Can you work these out from the model? Positions are in its coordinate system, mm. Face numbers are marked on the shaded views. A direction names the side the tool comes from. Give positions to 0.01 mm unless a question says otherwise; leave off trailing zeros. Loops run counter-clockwise (first coordinate to the right, second up) from the corner with the lowest first, then second, coordinate; pieces in that order, holes last. Notation, with made-up numbers: (-24, -35.75) -> (-7, -35.75) arc R12 cw to (-7, -25.75) -> close; hole circle Ø1 at (68.25, 38). An arc over 180 degrees is marked (long way). One line per question, with ' | ' between items.
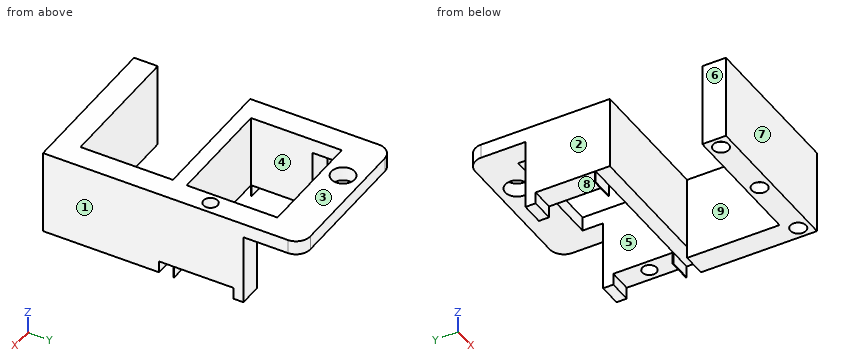
Autodesk Inventor part; units mm, degrees
ref_plane "Work Plane2" through (28, 0, 0) normal (0, 0, 1) x (1, 0, 0)
ref_plane "Work Plane3" through (0, -3.15, -2.5) normal (0, 0, 1) x (1, 0, 0)
ref_plane "YZ Plane" through (0, 0, 0) normal (1, 0, 0) x (0, 1, 0)
ref_plane "Work Plane1" through (5, 0, 4.5) normal (0, 0, 1) x (1, 0, 0)
sketch "Sketch1" plane through (5, 0, 4.5) normal (0, 0, 1) x (1, 0, 0)
  circle A0 centre (25.5, 6.25) radius 1.5
  line L0 (28, 14.65) -> (28, -27.65)
  line L1 (23.15, 14.65) -> (28, 14.65)
  line L2 (23.15, 14.65) -> (23.15, -0.15)
  line L3 (-0.15, -0.15) -> (23.15, -0.15)
  line L4 (-0.15, 14.65) -> (-0.15, -0.15)
  line L5 (-5, 14.65) -> (-0.15, 14.65)
  line L6 (-5, 14.65) -> (-5, -3.15)
  line L7 (23, -3.15) -> (-5, -3.15)
  circle A1 centre (25.5, -25.15) radius 1.5
  circle A2 centre (-2.5, -25.15) radius 1.5
  circle A3 centre (11.5, -25.15) radius 1.5
  line L8 (23, -22.65) -> (23, -3.15)
  line L9 (23, -22.65) -> (-5, -22.65)
  line L10 (-5, -22.65) -> (-5, -27.65)
  line L11 (28, -27.65) -> (-5, -27.65)
  point P0 (-5, 0)
ref_plane "Work Plane2" through (28, 0, 0) normal (0, 0, 1) x (1, 0, 0)
extrude "Extrusion1" add sketch "Sketch1" against normal up to surface (4.5 mm away) contours L0 L11 L10 L9 L8 L7 L6 L5 L4 L3 L2 L1 | A1 | A2 | A3
sketch "Sketch2" plane through (33, -3.15, 0) normal (0, 0, -1) x (-1, 0, 0)
  circle A0 centre (2.5, 9.4) radius 1.5
  line L0 (4.85, 17.8) -> (0, 17.8)
  line L1 (0, 17.8) -> (0, -24.5)
  line L2 (5, 0) -> (33, 0)
  line L3 (33, 0) -> (33, 17.8)
  line L4 (33, 17.8) -> (28.15, 17.8)
  line L5 (28.15, 17.8) -> (28.15, 3)
  line L6 (28.15, 3) -> (4.85, 3)
  line L7 (4.85, 3) -> (4.85, 17.8)
  line L8 (5, 15.65) -> (0, 15.65)
  line L9 (5, 3.15) -> (0, 3.15)
  line L10 (33, 15.65) -> (28, 15.65)
  line L11 (33, 3.15) -> (28, 3.15)
  line L12 (0, 17.8) -> (4.85, 17.8)
  line L13 (4.85, 17.8) -> (4.85, 3)
  line L14 (0, 17.8) -> (4.85, 17.8)
  line L15 (4.85, 17.8) -> (4.85, 15.65)
  line L16 (4.85, 15.65) -> (0, 15.65)
  line L17 (0, 15.65) -> (0, 17.8)
  line L18 (28.15, 17.8) -> (33, 17.8)
  line L19 (33, 17.8) -> (33, 15.65)
  line L20 (33, 15.65) -> (28.15, 15.65)
  line L21 (28.15, 15.65) -> (28.15, 17.8)
  line L22 (33, 0) -> (5, 0)
  line L23 (0, -24.5) -> (0, 17.8)
  line L24 (33, 0) -> (0, 0)
  line L25 (0, 0) -> (0, 3)
  line L26 (0, 3) -> (33, 3)
  line L27 (33, 3) -> (33, 0)
  line L28 (28.15, 3.15) -> (33, 3.15)
  line L29 (33, 3.15) -> (33, 3)
  line L30 (33, 3) -> (28.15, 3)
  line L31 (28.15, 3) -> (28.15, 3.15)
  line L32 (4.85, 3.15) -> (0, 3.15)
  line L33 (0, 3.15) -> (0, 3)
  line L34 (0, 3) -> (4.85, 3)
  line L35 (4.85, 3) -> (4.85, 3.15)
  line L36 (0, -24.5) -> (33, -24.5)
  line L37 (33, -24.5) -> (33, -19.5)
  line L38 (33, -19.5) -> (5, -19.5)
  line L39 (5, -19.5) -> (5, 0)
ref_plane "Work Plane3" through (0, -3.15, -2.5) normal (0, 0, 1) x (1, 0, 0)
extrude "Extrusion2" add sketch "Sketch2" along normal up to surface (2.5 mm away) contours L7 L8 L1 L0 | L7 L26 L1 L9 | L5 L11 L3 L26 | L5 L4 L3 L10
ref_plane "Work Plane5" through (11.25, 23, 12.45) normal (0, 0, 1) x (-1, 0, 0)
sketch "Sketch4" plane through (11.25, 23, 12.45) normal (0, 0, 1) x (-1, 0, 0)
  circle A0 centre (0, 0) radius 2.45
  arc A1 (-21.75, -1) -> (-18.75, -4) centre (-18.75, -1) ccw
  line L0 (8.25, -4) -> (-18.75, -4)
  arc A2 (8.25, -4) -> (11.25, -1) centre (8.25, -1) ccw
  line L1 (11.25, 5.35) -> (11.25, -1)
  line L2 (6.4, 5.35) -> (11.25, 5.35)
  line L3 (6.4, 4) -> (6.4, 5.35)
  line L4 (-16.9, 4) -> (6.4, 4)
  line L5 (-16.9, 5.35) -> (-16.9, 4)
  line L6 (-21.75, 5.35) -> (-16.9, 5.35)
  line L7 (-21.75, -1) -> (-21.75, 5.35)
  point P0 (11.25, 23)
extrude "Extrusion3" add sketch "Sketch4" along normal blind 3
sketch "Sketch5" plane through (11.25, 23, 15.45) normal (0, 0, 1) x (1, 0, 0)
  line L0 (-6.4, -5.35) -> (-11.25, -5.35)
  line L1 (-6.4, -8.35) -> (-11.25, -8.35)
  line L2 (-11.25, -5.35) -> (-6.4, -5.35)
  line L3 (-6.4, -5.35) -> (-6.4, -8.35)
  line L4 (-6.4, -8.35) -> (-11.25, -8.35)
  line L5 (-11.25, -8.35) -> (-11.25, -5.35)
  line L6 (16.9, -5.35) -> (21.75, -5.35)
  line L7 (21.75, -8.35) -> (16.9, -8.35)
  line L8 (16.9, -5.35) -> (21.75, -5.35)
  line L9 (21.75, -5.35) -> (21.75, -8.35)
  line L10 (21.75, -8.35) -> (16.9, -8.35)
  line L11 (16.9, -8.35) -> (16.9, -5.35)
  circle A0 centre (19.25, -16.75) radius 1.5
  line L12 (21.75, -50.65) -> (21.75, -8.35)
  line L13 (21.75, -8.35) -> (16.9, -8.35)
  line L14 (16.9, -8.35) -> (16.9, -23.15)
  line L15 (16.9, -23.15) -> (-6.4, -23.15)
  line L16 (-6.4, -23.15) -> (-6.4, -8.35)
  line L17 (-6.4, -8.35) -> (-11.25, -8.35)
  line L18 (-11.25, -8.35) -> (-11.25, -26.15)
  line L19 (-11.25, -26.15) -> (16.75, -26.15)
  line L20 (16.75, -26.15) -> (16.75, -45.65)
  line L21 (16.75, -45.65) -> (-11.25, -45.65)
  line L22 (-11.25, -45.65) -> (-11.25, -50.65)
  line L23 (-11.25, -50.65) -> (21.75, -50.65)
  point P0 (-11.25, -23)
extrude "Extrusion4" add sketch "Sketch5" against normal blind 3
sketch "Sketch6" plane through (5, 0, 4.5) normal (0, 0, 1) x (1, 0, 0)
  line L0 (-5, 14.65) -> (-0.15, 14.65)
  circle A0 centre (25.5, 6.25) radius 1.5
  line L1 (28, 14.65) -> (28, -27.65)
  line L2 (23.15, 14.65) -> (28, 14.65)
  line L3 (23.15, 14.65) -> (23.15, -0.15)
  line L4 (-0.15, -0.15) -> (23.15, -0.15)
  line L5 (-0.15, 14.65) -> (-0.15, -0.15)
  line L6 (-5, 14.65) -> (-0.15, 14.65)
  line L7 (-5, 14.65) -> (-5, -3.15)
  line L8 (23, -3.15) -> (-5, -3.15)
  circle A1 centre (6.25, 23) radius 10
  circle A2 centre (6.25, 23) radius 12
  line L9 (-2.3684, 14.65) -> (-5, 14.65)
  line L10 (-5, 12.5) -> (-5, 14.65)
  line L11 (-5, 14.65) -> (-5, 12.5)
  line L12 (-0.15, 12.5) -> (-5, 12.5)
  line L13 (-5, 12.5) -> (-0.15, 12.5)
  line L14 (-0.15, 12.5) -> (-0.15, 12.8491)
  line L15 (-0.15, 14.65) -> (-0.15, 12.5)
  circle A3 centre (25.5, -25.15) radius 1.5
  circle A4 centre (-2.5, -25.15) radius 1.5
  circle A5 centre (11.5, -25.15) radius 1.5
  line L16 (23, -22.65) -> (23, -3.15)
  line L17 (23, -22.65) -> (-5, -22.65)
  line L18 (-5, -22.65) -> (-5, -27.65)
  line L19 (28, -27.65) -> (-5, -27.65)
  point P0 (-5, 0)
  dimension "d8" = 2
extrude "Extrusion5" add sketch "Sketch6" along normal up to surface (7.95 mm away) contours L0 A2 L5 L12 L7 | L12 L5 L4 L3 L2 L1 L19 L18 L17 L16 L8 L7 | A3 | A4 | A5
sketch "Sketch7" plane through (33, 0, 0) normal (1, 0, 0) x (0, 0, -1)
  line L0 (-15.45, -3.15) -> (0, -3.15)
  line L1 (-15.45, -3.15) -> (2.5, -3.15)
  line L2 (2.5, -3.15) -> (2.5, -22.65)
  line L3 (2.5, -22.65) -> (-15.45, -22.65)
  line L4 (-15.45, -22.65) -> (-15.45, -3.15)
  line L5 (-15.45, 4.75) -> (0, 4.75)
  line L6 (-12.45, 24) -> (-12.45, 14.65)
  line L7 (-12.45, 24) -> (-15.45, 24)
  line L8 (-15.45, 24) -> (-15.45, -27.65)
  line L9 (2.5, 0) -> (2.5, -0.15)
  line L10 (0, 0) -> (2.5, 0)
  line L11 (0, 12.5) -> (0, 0)
  line L12 (0, 12.5) -> (2.5, 12.5)
  line L13 (2.5, 14.65) -> (2.5, 12.5)
  line L14 (-12.45, 14.65) -> (2.5, 14.65)
  line L15 (-15.45, -22.65) -> (2.5, -22.65)
  line L16 (2.5, -22.65) -> (2.5, -27.65)
  line L17 (2.5, -27.65) -> (-15.45, -27.65)
  line L18 (-15.45, -27.65) -> (-15.45, -22.65)
  line L19 (0, -0.15) -> (0, -27.65)
  line L20 (0, -0.15) -> (2.5, -0.15)
  line L21 (-15.45, -27.65) -> (0, -27.65)
  point P0 (0, 0)
  point P1 (2.5, -3.15)
  dimension "d11" = 19.5
  dimension "d13" = 5
extrude "Extrusion6" add sketch "Sketch7" against normal blind 5 contours L0 L19 L3 L4 | L1 L2 L3 L19 | L3 L19 L17 L8 | L3 L16 L17 L19
extrude "Extrusion7" add sketch "Sketch7" against normal up to surface (33 mm away) contours L3 L19 L17 L8 | L3 L16 L17 L19
sketch "Sketch8" plane through (33, -27.65, -2.5) normal (0, 0, -1) x (-1, 0, 0)
  circle A0 centre (2.5, 2.5) radius 1.65
  circle A1 centre (16.5, 2.5) radius 1.65
  circle A2 centre (30.5, 2.5) radius 1.65
  line L0 (2.5, 2.5) -> (16.5, 2.5) construction
  line L1 (16.5, 2.5) -> (30.5, 2.5) construction
  line L2 (0, 0) -> (33, 0) construction
  line L3 (0, 0) -> (0, 24.5) construction
  line L4 (33, 0) -> (33, 5) construction
  point P0 (33, 27.65)
  dimension "d18" = 3.3
  dimension "d19" = 3.3
  dimension "d20" = 3.3
  dimension "d21" = 2.5
  dimension "d22" = 2.5
  dimension "d23" = 2.5
extrude "Extrusion8" cut sketch "Sketch8" against normal blind 2.5
properties part number "Bracket 2"
Q1. On a 3-axis mill with a long thin cutter (end or side, diameter ignored), from which of +Z, -Z, +X, -X, +Y, -Y can I reach the whole of each face in a straight line? I mean the marked faces 5, 6, 7, 8 and 9. Say none if no direction works.
Entries:
face 5: +Z, -Z | face 6: +Z, -Z, -X, +Y, -Y | face 7: +Z, -Z, +X, -X, -Y | face 8: -Z, +X, -X | face 9: +Z, -Z, -X
Q2. If we section it at D-D (x = 13): Write out the boundary of the cut face in (y, z).
Entries:
outline: (-27.65, -2.5) -> (-22.65, -2.5) -> (-22.65, 15.45) -> (-27.65, 15.45) -> close; (-3.15, 0) -> (-0.15, 0) -> (-0.15, 15.45) -> (-3.15, 15.45) -> close; (19, 12.45) -> (21.29, 12.45) -> (21.29, 15.45) -> (19, 15.45) -> close; (24.71, 12.45) -> (27, 12.45) -> (27, 15.45) -> (24.71, 15.45) -> close
Q3. If we mould it in two halves opening along X, with no side actions, what happens to the marked faces 1, 2, 3 and 4? For each: pulls with the +X half, pulls with the -X half, needs draft (parallel to the pull), parting line crosses it, or undercut.
Entries:
face 1: pulls with the +X half | face 2: pulls with the -X half | face 3: needs draft | face 4: undercut
Q4. If we section it at A-A (y = 6.25): Write out the boundary of the cut face in (x, z).
Entries:
outline: (0, 0) -> (4.85, 0) -> (4.85, 15.45) -> (0, 15.45) -> close; (28.15, 0) -> (29, 0) -> (29, 15.45) -> (28.15, 15.45) -> close; (32, 0) -> (33, 0) -> (33, 15.45) -> (32, 15.45) -> close
Q5. If I drill on probe 1 along Y at (x, z) = (2.5, -0.85); probe 2 along Y at (x, z) = (30.5, -0.7); probe 3 along Y at (x, z) = (26.5, 14), over which ranges is the centre line in solid material (lowest first)? Write a range as from..to.
Entries:
probe 1: -27.65..-26.8, -23.5..-22.65, -0.15..0, 12.5..14.65 | probe 2: -27.65..-26.8, -23.5..-3.15, -0.15..0, 12.5..14.65 | probe 3: -27.65..-22.65, -3.15..-0.15, 19..27
Q6. If we section it at C-C (y = 23): Write out the boundary of the cut face in (x, z).
Entries:
outline: (0, 12.45) -> (8.8, 12.45) -> (8.8, 15.45) -> (0, 15.45) -> close; (13.7, 12.45) -> (33, 12.45) -> (33, 15.45) -> (13.7, 15.45) -> close
Q7. If we section it at B-B (x = 25): Write out the boundary of the cut face in (y, z).
Entries:
outline: (-27.65, -2.5) -> (-22.65, -2.5) -> (-22.65, 15.45) -> (-27.65, 15.45) -> close; (-3.15, 0) -> (-0.15, 0) -> (-0.15, 15.45) -> (-3.15, 15.45) -> close; (19, 12.45) -> (27, 12.45) -> (27, 15.45) -> (19, 15.45) -> close
Q8. For pin 1 Ø2 at (y, z) = (16.5, 6) entering from -X; pin 2 Ø1.5 at (x, z) = (26, 6) entering from +Y; pin 3 Ø0.9 at (x, y) = (19, -2.5) entering from -Z; pin 4 Ø2 at (x, z) = (31.5, -1.5) entering from +Y, each with a flat end and sliding along its axis, tell me the tip position at first contact or that it passes through.
Entries:
pin 1: through | pin 2: y = -0.15 | pin 3: z = 0 | pin 4: y = 14.65
